Source: CAD feature listing. Evaluate the final solid. Frame: model axes, mm. A direction names the side the tool comes from. Coordinates: 2 decimals unless noted, no trailing zeros. Loops run counter-clockwise (first coordinate to the right, second up) from the corner with the lowest first, then second, coordinate; pieces in that order, holes last.
from build123d import *

# Parameters (mm, degrees)
F0_W     = 70
F0_H     = 50
F0_W_2   = 8
F0_H_2   = 2.962767
F0_H_3   = 3
F1_DEPTH = 3


with BuildPart() as f1:
    # F0 (on Top) → F1 (new body)
    with BuildSketch(Plane.XY):
        with Locations((0, 0.110523)):
            Rectangle(F0_W, F0_H)
        with Locations((-17, -20.408093)):
            Rectangle(F0_W_2, F0_H_2, mode=Mode.SUBTRACT)
        with Locations((17, -20.389477)):
            Rectangle(F0_W_2, F0_H_3, mode=Mode.SUBTRACT)
        with BuildLine():
            ThreePointArc((-19.451462, -1.499214), (-20.999804, -0.024272), (-19.5, 1.5))
            Line((-19.5, 1.5), (-0.362987, 3.490252))
            Line((-0.362987, 3.490252), (0, 3.528003))
            Line((0, 3.528003), (19.654556, 1.492016))
            ThreePointArc((19.654556, 1.492016), (20.613964, 1.004531), (21, 0))
            ThreePointArc((21, 0), (20.543358, -1.077684), (19.451462, -1.499214))
            Line((19.451462, -1.499214), (0.364042, -3.490142))
            Line((0.364042, -3.490142), (0, -3.528114))
            Line((0, -3.528114), (-0.364042, -3.490142))
            Line((-0.364042, -3.490142), (-19.451462, -1.499214))
        make_face(mode=Mode.SUBTRACT)
    extrude(amount=F1_DEPTH)


solid = f1.part
Q1. Draft query along Y for faces 1 (the flat face through (35, 0, 1)), 2 (the flat face through (0, -24.889, 1)), 3 (the cylindrical face through (-21, 0, 1)), 4 (the flat face through (9.69, 2.524, 1.479)). Return one class per face: +Y half, -Y half, draft (parallel to the pull), parting line (faces both ways), or undercut.
Q2. Section A-A, the plane z = 2.3. Return the cut outline in (x, y).
Q3. Section D-D, the plane x = 5. Return the cut outline in (y, z).
Q4. Access query for faces 5 (the flat face through (0, 25.111, 1)), 6 (the flat face through (21, -20, 1)). Directions: +Z, -Z, +X, -X, +Y, -Y. A direction counts if a zero-diameter tool reaches every point of the face in a straight line with its end or side. Return the directions, or none.
Q5. Section B-B, the plane x = -2. Return the cut outline in (y, z).
Q6. Section C-C, the plane x = 14. Return the cut outline in (y, z), plus the area to 3 significant figures.
Q7. Line query: line 1 along X through (y, z) = (-21, 0.75); line 2 along Y through (x, z) = (16.5, 1.5); line 3 along Y through (x, z) = (20.5, 1.25). Output: solid intervals per line, ascending.
Derived:
1. face 1: draft
1. face 2: -Y half
1. face 3: undercut
1. face 4: undercut
2. outline: (-35, -24.89) - (35, -24.89) - (35, 25.11) - (-35, 25.11) - close; hole (-21, -21.89) - (-13, -21.89) - (-13, -18.93) - (-21, -18.93) - close; hole (-19.5, 1.5) arc R1.5 ccw (long way) to (-19.45, -1.5) - (-0.36, -3.49) - (0, -3.53) - (0.36, -3.49) - (19.45, -1.5) arc R1.5 ccw to (21, 0) arc R1.5 ccw to (19.65, 1.49) - (0, 3.53) - (-0.36, 3.49) - close; hole (13, -21.89) - (21, -21.89) - (21, -18.89) - (13, -18.89) - close
3. outline: (-24.89, 0) - (-3.01, 0) - (-3.01, 3) - (-24.89, 3) - close; (3.01, 0) - (25.11, 0) - (25.11, 3) - (3.01, 3) - close
4. face 5: +Z, -Z, +X, -X, +Y
4. face 6: +Z, -Z
5. outline: (-24.89, 0) - (-3.32, 0) - (-3.32, 3) - (-24.89, 3) - close; (3.32, 0) - (25.11, 0) - (25.11, 3) - (3.32, 3) - close
6. outline: (-24.89, 0) - (-21.89, 0) - (-21.89, 3) - (-24.89, 3) - close; (-18.89, 0) - (-2.07, 0) - (-2.07, 3) - (-18.89, 3) - close; (2.08, 0) - (25.11, 0) - (25.11, 3) - (2.08, 3) - close
6. area: 129 mm2
7. line 1: x = -35 to -21, -13 to 13, 21 to 35
7. line 2: y = -24.89 to -21.89, -18.89 to -1.81, 1.82 to 25.11
7. line 3: y = -24.89 to -21.89, -18.89 to -1.12, 1.12 to 25.11
